Autodesk Inventor part; units mm, degrees
ref_plane "YZ Plane" through (0, 0, 0) normal (1, 0, 0) x (0, 1, 0)
ref_plane "XZ Plane" through (0, 0, 0) normal (0, 1, 0) x (-1, 0, 0)
ref_plane "XY Plane" through (0, 0, 0) normal (0, 0, 1) x (1, 0, 0)
sketch "Skizze1" plane through (0, 0, 0) normal (0, 1, 0) x (-1, 0, 0)
  line L0 (10, 0) -> (90, 0)
  line L1 (100, 0) -> (100, -116)
  line L2 (100, -116) -> (0, -116)
  line L3 (0, -116) -> (0, 0)
  line L4 (100, 0) -> (90, 0)
  line L5 (90, 0) -> (90, 2)
  line L6 (90, 2) -> (100, 2)
  line L7 (100, 2) -> (100, 0)
  line L8 (0, 0) -> (10, 0)
  line L9 (10, 0) -> (10, 2)
  line L10 (10, 2) -> (0, 2)
  line L11 (0, 2) -> (0, 0)
  dimension "d0" = 116
  dimension "d1" = 100
  dimension "d58" = 10
  dimension "d59" = 2
  dimension "d60" = 10
  dimension "d61" = 2
extrude "Extrusion1" add sketch "Skizze1" along normal blind 1.6
sketch "Skizze2" plane through (0, 1.6, 0) normal (0, 1, 0) x (1, 0, 0)
  line L0 (0, 116) -> (-100, 116)
  line L1 (-100, 116) -> (-100, -2)
  point P0 (0, 0)
  point P1 (-95, 111)
  point P2 (-100, 0)
  dimension "d4" = 5
  dimension "d5" = 5
hole "Bohrung1" at (-95, 1.6, -111) direction (0, -1, 0) diameter 3.5 end through all
pattern_linear "Rechteckige Anordnung1" count 2 spacing 109 along (0, 0, 1) count 2 spacing 90 along (1, 0, 0) of "Bohrung1"
sketch "Skizze3" plane through (0, 1.6, 0) normal (0, 1, 0) x (1, 0, 0)
  line L0 (-98.5, 8.5) -> (-94.5, 8.5)
  line L1 (-94.5, 8.5) -> (-94.5, 105.5)
  line L2 (-94.5, 105.5) -> (-98.5, 105.5)
  line L3 (-98.5, 105.5) -> (-98.5, 8.5)
  line L4 (-100, 116) -> (-100, -2)
  line L5 (0, 116) -> (-100, 116)
  line L6 (-94, 50.5) -> (-73, 50.5)
  line L7 (-73, 50.5) -> (-73, 54.5)
  line L8 (-73, 54.5) -> (-94, 54.5)
  line L9 (-94, 54.5) -> (-94, 50.5)
  line L10 (-72.5, 110.5) -> (-29.5, 110.5)
  line L11 (-29.5, 110.5) -> (-29.5, 114.5)
  line L12 (-29.5, 114.5) -> (-72.5, 114.5)
  line L13 (-72.5, 114.5) -> (-72.5, 110.5)
  line L14 (-28, 56) -> (-24, 56)
  line L15 (-24, 56) -> (-24, 89)
  line L16 (-24, 89) -> (-28, 89)
  line L17 (-28, 89) -> (-28, 56)
  line L18 (0, 0) -> (0, 116)
  line L19 (-67.5, 50.5) -> (-62.5, 50.5)
  line L20 (-62.5, 50.5) -> (-62.5, 66.5)
  line L21 (-62.5, 66.5) -> (-67.5, 66.5)
  line L22 (-67.5, 66.5) -> (-67.5, 50.5)
  line L23 (-71, 48.5) -> (-96, 48.5)
  line L24 (-96, 48.5) -> (-96, 56.5)
  line L25 (-96, 56.5) -> (-71, 56.5)
  line L26 (-71, 56.5) -> (-71, 48.5)
  line L27 (-92.5, 107.5) -> (-92.5, 6.5)
  line L28 (-92.5, 6.5) -> (-100.5, 6.5)
  line L29 (-100.5, 6.5) -> (-100.5, 107.5)
  line L30 (-100.5, 107.5) -> (-92.5, 107.5)
  line L31 (-69.5, 48.5) -> (-60.5, 48.5)
  line L32 (-60.5, 48.5) -> (-60.5, 68.5)
  line L33 (-60.5, 68.5) -> (-69.5, 68.5)
  line L34 (-69.5, 68.5) -> (-69.5, 48.5)
  line L35 (-27.5, 108.5) -> (-74.5, 108.5)
  line L36 (-74.5, 108.5) -> (-74.5, 116.5)
  line L37 (-74.5, 116.5) -> (-27.5, 116.5)
  line L38 (-27.5, 116.5) -> (-27.5, 108.5)
  line L39 (-30, 54) -> (-22, 54)
  line L40 (-22, 54) -> (-22, 91)
  line L41 (-22, 91) -> (-30, 91)
  line L42 (-30, 91) -> (-30, 54)
  point P0 (-100, 0)
  point P1 (-27.5, 116)
  point P2 (-74.5, 116)
  point P3 (-92.5, 48.5)
  point P4 (-92.5, 56.5)
  point P5 (-100, 107.5)
  point P6 (-100, 6.5)
  dimension "d19" = 97
  dimension "d20" = 4
  dimension "d21" = 1.5
  dimension "d22" = 10.5
  dimension "d23" = 4
  dimension "d24" = 21
  dimension "d25" = 61.5
  dimension "d26" = 6
  dimension "d27" = 43
  dimension "d28" = 4
  dimension "d29" = 1.5
  dimension "d30" = 27.5
  dimension "d31" = 4
  dimension "d32" = 33
  dimension "d33" = 24
  dimension "d34" = 27
  dimension "d47" = 5
  dimension "d48" = 16
  dimension "d49" = 0
  dimension "d50" = 62.5
  dimension "d53" = 2
  dimension "d54" = 2
  dimension "d55" = 2
  dimension "d56" = 2
  dimension "d57" = 2
extrude "Extrusion2" cut sketch "Skizze3" against normal through all contours L3 L2 L1 L25 L24 L23 L0 | L0 L1 L23 L27 L28 L4 L30 L25 L2 L3 | L23 L24 L25 L1 | L1 L25 L27 L8 L9 L6 L23 | L27 L6 L7 L8 L25 L26 L23 | L5 L38 L35 L36 | L27 L8 L7 L6 | L6 L9 L8 L27 | L13 L12 L11 L10 | L17 L16 L15 L14 | L22 L21 L20 L19 | L34 L33 L32 L31 | L42 L41 L40 L39
fillet "Rundung1" radius 1 28 edges at (-100, 0.8, 2) (-100, 0.8, -116) (-74.5, 0.8, -116) (-74.5, 0.8, -108.5) (-69.5, 0.8, -68.5) (-60.5, 0.8, -68.5) (-60.5, 0.8, -48.5) (-69.5, 0.8, -48.5) (-71, 0.8, -56.5) (-71, 0.8, -48.5) (-92.5, 0.8, -56.5) (-92.5, 0.8, -48.5) (-90, 0.8, 0) (-90, 0.8, 2) (-92.5, 0.8, -6.5) (-100, 0.8, -6.5) (-10, 0.8, 2) (-10, 0.8, 0) (0, 0.8, 2) (-22, 0.8, -54) (-30, 0.8, -54) (-30, 0.8, -91) (-22, 0.8, -91) (-27.5, 0.8, -108.5) (-27.5, 0.8, -116) (0, 0.8, -116) (-92.5, 0.8, -107.5) (-100, 0.8, -107.5)
sketch "Skizze4" plane through (0, 1.6, 0) normal (0, 1, 0) x (1, 0, 0)
  circle A0 centre (-45, 76) radius 2
  line L0 (-1, 116) -> (-26.5, 116)
  line L1 (0, -1) -> (0, 115)
  circle A1 centre (-33.5, 55) radius 2
  line L2 (-52, 60.5) -> (-45, 60.5) construction
  line L3 (-52, 58.5) -> (-45, 58.5)
  line L4 (-45, 62.5) -> (-52, 62.5)
  arc A2 (-52, 62.5) -> (-52, 58.5) centre (-52, 60.5) ccw
  arc A3 (-45, 58.5) -> (-45, 62.5) centre (-45, 60.5) ccw
  line L5 (-75.5, 116) -> (-99, 116)
  line L6 (-100, 115) -> (-100, 108.5)
  circle A4 centre (-46, 38.5) radius 3
  circle A5 centre (-35, 38.5) radius 3
  line L7 (-9, -2) -> (-1, -2)
  line L8 (-64, 17) -> (-64, 36) construction
  line L9 (-62, 17) -> (-62, 36)
  line L10 (-66, 36) -> (-66, 17)
  arc A6 (-66, 17) -> (-62, 17) centre (-64, 17) ccw
  arc A7 (-62, 36) -> (-66, 36) centre (-64, 36) ccw
  line L11 (-100, 5.5) -> (-100, -1)
  line L12 (-64, 36) -> (-69, 36) construction
  line L13 (-64, 38) -> (-69, 38)
  line L14 (-69, 34) -> (-64, 34)
  arc A8 (-64, 34) -> (-64, 38) centre (-64, 36) ccw
  arc A9 (-69, 38) -> (-69, 34) centre (-69, 36) ccw
  circle A10 centre (-45, 16) radius 1.5
  point P0 (0, 0)
  point P1 (-48.5, 60.5)
  point P2 (-64, 26.5)
  point P3 (-66.5, 36)
  dimension "d63" = 4
  dimension "d64" = 40
  dimension "d65" = 45
  dimension "d66" = 4
  dimension "d67" = 33.5
  dimension "d68" = 61
  dimension "d69" = 7
  dimension "d70" = 4
  dimension "d71" = 55.5
  dimension "d72" = 48
  dimension "d73" = 6
  dimension "d74" = 6
  dimension "d75" = 11
  dimension "d76" = 0
  dimension "d77" = 35
  dimension "d79" = 77.5
  dimension "d80" = 19
  dimension "d81" = 4
  dimension "d82" = 36
  dimension "d83" = 80
  dimension "d84" = 5
  dimension "d85" = 4
  dimension "d86" = 3
  dimension "d87" = 100
  dimension "d88" = 45
extrude "Ausklinkung1" cut sketch "Skizze4" against normal blind 2
equation "\"Biegeradius\" = Stärke"
equation "\"BreiteBiegungsfreistellung\" = Stärke"
equation "\"TiefeBiegungsfreistellung\" = 0.5 * Stärke"
equation "\"GrößeEckenfreistellung\" = 4 * Stärke"
equation "\"MinimalRest\" = 2 * Stärke"
equation "\"Übergangsradius\" = Biegeradius"
equation "\"JacobiRadiusGröße\" = Biegeradius"
equation "\"Abstandsgröße\" = Stärke"
equation "\"d89\" = Stärke"
properties part number "mainunitshield"
Geometry check sheet. Reference: the model listing, model coordinates, mm. Round coordinates to 2 decimals unless told otherwise and drop trailing zeros. Order: outer loops, then holes, each group sorted by start corner. A loop starts at its lowest first (then second) coordinate and runs counter-clockwise, first axis right, second up. Notation, with made-up numbers: (-12.75, 69) - (32.25, 69) arc R28 ccw to (32.25, 91) - close; hole circle Ø10 at (-26.5, 68). An arc over 180 degrees is marked (long way). One line per question, with ' | ' between items. Start each with the question number.
(1) Sectioned sample at A-A on z = -23.5. Record the cut outline in (x, y).
(2) Sectioned sample at B-B on z = -111. Record the cut outline in (x, y).
(3) Thickness scan on L1, parallel to X at y = 0.9, z = -2; L2, parallel to X at y = 0.55, z = -111; L3, parallel to X at y = 0.3, z = -76. Record the ranges inside material, lowest first. Write a range as [from, to].
(4) Sectioned sample at D-D on z = -64. Record the cut outline in (x, y).
(5) Sectioned sample at C-C on x = -95. Record the cut outline in (y, z).
(6) Depth check by flat-ended pin: pin 1 Ø0.5 at (x, y) = (-25, 0.5) entering from +Z; pin 2 Ø0.5 at (y, z) = (1, -61.5) entering from -X; pin 3 Ø0.5 at (x, y) = (-58, 0.5) entering from -Z. Enter the tip coordinate at first touch or a pass-through.
(7) Release check for a two-part mould opening along X. For faces 1 (the flat face through (-49, 1.6, -56)), 2 (the cylindrical face through (-48.21, 0.81, -40.53)) record: released by +X, released by -X, zero draft, split by the parting line, or undercut.
Conclusion:
1) outline: (-92.5, 0) - (-66, 0) - (-66, 1.6) - (-92.5, 1.6) - close; (-62, 0) - (0, 0) - (0, 1.6) - (-62, 1.6) - close
2) outline: (-100, 0) - (-96.75, 0) - (-96.75, 1.6) - (-100, 1.6) - close; (-93.25, 0) - (-74.5, 0) - (-74.5, 1.6) - (-93.25, 1.6) - close; (-27.5, 0) - (-6.75, 0) - (-6.75, 1.6) - (-27.5, 1.6) - close; (-3.25, 0) - (0, 0) - (0, 1.6) - (-3.25, 1.6) - close
3) L1: x = [-100, -96.75], [-93.25, -6.75], [-3.25, 0] | L2: x = [-100, -96.75], [-93.25, -74.5], [-27.5, -6.75], [-3.25, 0] | L3: x = [-92.5, -47], [-43, -30], [-22, 0]
4) outline: (-92.5, 0) - (-69.5, 0) - (-69.5, 1.6) - (-92.5, 1.6) - close; (-60.5, 0) - (-30, 0) - (-30, 1.6) - (-60.5, 1.6) - close; (-22, 0) - (0, 0) - (0, 1.6) - (-22, 1.6) - close
5) outline: (0, -116) - (1.6, -116) - (1.6, -112.75) - (0, -112.75) - close; (0, -109.25) - (1.6, -109.25) - (1.6, -107.5) - (0, -107.5) - close; (0, -6.5) - (1.6, -6.5) - (1.6, -3.75) - (0, -3.75) - close; (0, -0.25) - (1.6, -0.25) - (1.6, 2) - (0, 2) - close
6) pin 1: stops at z = 0 | pin 2: stops at x = -92.5 | pin 3: stops at z = -108.5
7) face 1: zero draft | face 2: undercut
